Work out the finished part from the listing and answer in its coordinate system (mm). Face numbers are marked on the shaded views. A direction names the side the tool comes from. Round coordinates to 2 decimals unless told otherwise and drop trailing zeros. Loops run counter-clockwise (first coordinate to the right, second up) from the corner with the lowest first, then second, coordinate; pieces in that order, holes last. Notation, with made-up numbers: M -39,58 L -2,58 A21 ccw -2,68 Z; hole C 20,16.25 d9. An arc over 180 degrees is marked long. One line per item, written item: value.
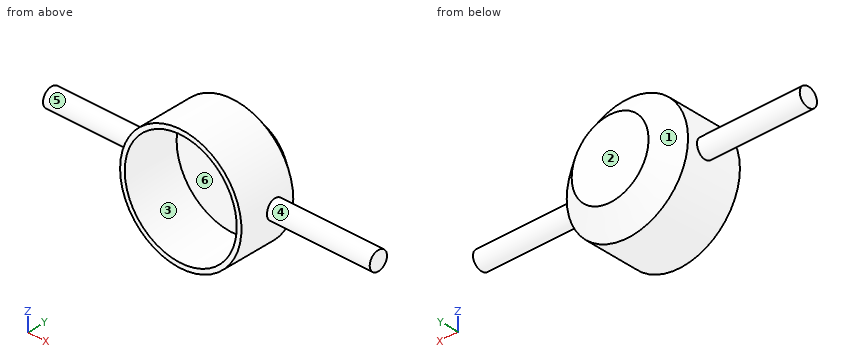
Autodesk Inventor part; units mm, degrees
ref_plane "Work Plane2" through (75.376, -18.8821, -44.9646) normal (1, 0, 0) x (0, 1, 0)
ref_plane "YZ Plane" through (0, 0, 0) normal (1, 0, 0) x (0, 1, 0)
ref_plane "XZ Plane" through (0, 0, 0) normal (0, 1, 0) x (-1, 0, 0)
sketch "Sketch1" plane through (0, 0, 0) normal (0, 1, 0) x (-1, 0, 0)
  circle A0 centre (0, 0) radius 152.4
  circle A1 centre (0, 0) radius 165.1
  dimension "d0" = 304.8
  dimension "d1" = 330.2
extrude "Extrusion1" add sketch "Sketch1" along normal blind 152.4
sketch "Sketch2" plane through (0, 0, 0) normal (1, 0, 0) x (0, 1, 0)
  circle A0 centre (100.6077, 0) radius 25.4
  point P0 (0, 0)
  dimension "d4" = 50.8
extrude "Extrusion2" add sketch "Sketch2" along normal mid plane 889
sketch "Sketch4" plane through (0, 152.4, 0) normal (0, 1, 0) x (1, 0, 0)
  circle A0 centre (0, 0) radius 152.4
extrude "Extrusion4" cut sketch "Sketch4" against normal through all
sketch "Sketch5" plane through (0, 152.4, 0) normal (0, 1, 0) x (1, 0, 0)
  circle A0 centre (0, 0) radius 165.1
extrude "Extrusion5" add sketch "Sketch5" along normal blind 50.8 draft -50
ref_plane "Work Plane2" through (75.376, -18.8821, -44.9646) normal (1, 0, 0) x (0, 1, 0)
sketch "Sketch9" plane through (75.376, -18.8821, -44.9646) normal (1, 0, 0) x (0, 1, 0)
  circle A0 centre (-604.603, 44.9646) radius 12.7
  point P0 (18.8821, 44.9646)
  dimension "d25" = 25.4
extrude "Extrusion9" cut sketch "Sketch9" against normal through all
properties part number "CapstanTop-ver1-1111-2021"
1) Find section A-A (z = 0). Give the vertices of the cut face in (x, y), then the cut area to 3 significant figures.
Check values:
outline: M -444.5,75.21 L -165.1,75.21 L -165.1,0 L -152.4,0 L -152.4,152.4 L 152.4,152.4 L 152.4,0 L 165.1,0 L 165.1,75.21 L 444.5,75.21 L 444.5,126.01 L 165.1,126.01 L 165.1,152.4 L 104.56,203.2 L -104.56,203.2 L -165.1,152.4 L -165.1,126.01 L -444.5,126.01 Z
area: 46,000 mm2
2) Find section B-B (x = 0). Give the vertices of the cut face in (y, z).
Check values:
outline: M 0,-165.1 L 152.4,-165.1 L 203.2,-104.56 L 203.2,104.56 L 152.4,165.1 L 0,165.1 L 0,152.4 L 152.4,152.4 L 152.4,-152.4 L 0,-152.4 Z
3) The mould has two halves that part along X. Classify the marked faces 1, 2 and 3: +X half, -X half, draft (parallel to the pull), parting line (faces both ways), or undercut.
Check values:
face 1: parting line
face 2: draft
face 3: undercut
4) Find the intervals of material crossed by probe 1 along X at (y, z) = (33.5, 0); probe 2 along X at (y, z) = (77, 0), in increasing order. Write a range as from..to.
Check values:
probe 1: -165.1..-152.4, 152.4..165.1
probe 2: -444.5..-152.4, 152.4..444.5
5) For the marked faces 4, 5 and 6, determine the directions among +Z, -Z, +X, -X, +Y, -Y from which every point of the face is accessible in a straight line to the end or side of a thin tool.
Check values:
face 4: +X
face 5: -X
face 6: -Y
6) Each of these flat-tipped pins is pushed along its axis until it touches: pin 1 (2 mm diameter, centred on y = 49, z = -71.5, fed in from +X); pin 2 (5 mm diameter, centred on y = 180.5, z = 109, fed in from +X); pin 3 (2 mm diameter, centred on y = 142, z = 117, fed in from +X). Where does it stop, or does it pass through?
Check values:
pin 1: x = 149.29
pin 2: x = 80
pin 3: x = 117.48
7) Find section C-C (y = 60). Give the vertices of the cut face in (x, z).
Check values:
outline: C 0,0 d330.2; hole C 0,0 d304.8
8) Find section D-D (x = -269). Give the vertices of the cut face in (y, z), then the cut area to 3 significant figures.
Check values:
outline: C 100.61,0 d50.8
area: 2,030 mm2
